For this review, take the finished solid that the model builds, in its own axes (mm). A direction names the side the tool comes from. Round coordinates to 2 decimals unless told otherwise and drop trailing zeros. Write each loop counter-clockwise with the first axis right and the second up, starting at its lowest first coordinate (ties: lowest second). Pieces come first, ordered by that corner, then holes. Notation, with made-up numbers: (38.5, 31.5) -> (71.5, 31.5) arc R21 ccw to (71.5, 67.5) -> close; hole circle Ø9 at (75, -22.75). An arc over 180 degrees is marked (long way). Answer as CSV lines item,"result". Start each with the question number.
Item 1: Mouldability with a two-part tool opening along Z and no side actions: class faces 4 (the flat face through (-31, 1.24, 30)), 5 (the flat face through (44, 1.95, -19)), 6 (the cylindrical face through (-44.339, -1.303, 29.796)), 7 (the flat face through (-44, -2, -7.6)) as +Z half, -Z half, draft (parallel to the pull), parting line (faces both ways), or undercut.
Item 2: Take a section at D-D on y = -3.25. Give the boundary of the cut face in (x, z), then the cut area to 3 significant figures.
Item 3: Take a section at B-B on x = -10. Give the boundary of the cut face in (y, z), then the cut area to 3 significant figures.
Item 4: Wall thickness on probe 1 along X at (y, z) = (-3, 21); probe 2 along Z at (x, y) = (9.5, -1.5); probe 3 along Z at (x, y) = (-20, 2): over which ranges is each line inside the solid? List them lowest first. Write a range as from..to.
Item 5: Take a section at A-A on z = -4. Give the boundary of the cut face in (x, y).
Item 6: Take a section at C-C on z = -19.5. Give the boundary of the cut face in (x, y), then the cut area to 3 significant figures.
Item 7: Machinability: for faces 1 (the flat face through (-44, -2, 7.4)), 2 (the flat face through (-41.05, -3, -17)), 3 (the cylindrical face through (-41.798, 1.232, -27.387)), which of the approach directions +Z, -Z, +X, -X, +Y, -Y give a long, thin tool a straight path to every point of the face, cutting with its end or side? Answer none if there is none.
Item 8: For pin 1 Ø4 at (x, z) = (-33, 30) entering from +Y; pin 2 Ø3 at (x, z) = (44.5, -4.5) entering from +Y; pin 3 Ø1.5 at (y, z) = (-3.5, -1) entering from -X, all flat-tipped, find the tip position at first contact; note any pin that passes through.
```python
from build123d import *

# Parameters (mm, degrees)
EXTRUDE_THIN1_DEPTH      = 2.5
EXTRUDE_THIN1_DEPTH_BACK = 5
EXTRUDE_THIN2_START      = -5
EXTRUDE_THIN2_DEPTH      = 5
CUT_EXTRUDE3_DEPTH       = 76.51403843
CUT_EXTRUDE3_DEPTH_BACK  = 1
CUT_EXTRUDE4_START       = -0.20682878
CUT_EXTRUDE4_OUTLINE_W   = 17
CUT_EXTRUDE4_OUTLINE_H   = 0.9
CUT_EXTRUDE4_OUTLINE_W_2 = 15.6
CUT_EXTRUDE4_OUTLINE_H_2 = 0.55
CUT_EXTRUDE4_DEPTH       = 3.80682878
SKETCH10_W               = 10
SKETCH10_H               = 15
CUT_EXTRUDE6_DEPTH       = 57.113902021
CUT_EXTRUDE11_DEPTH      = 95.199363055
CUT_EXTRUDE11_DEPTH_BACK = 5


# Read off the part's stored shape, not the designer's step: Cut-Extrude4
with BuildPart() as part:
    # Sketch1 → Extrude-Thin1 (new, two sides: drawn at the far end of the back side and taken through both)
    with BuildSketch(Plane(origin=(0, 0, 0), x_dir=(1, 0, 0), z_dir=(0, 1, 0)).offset(-EXTRUDE_THIN1_DEPTH_BACK)):
        with BuildLine():
            Line((-46.05, 25.6), (-46.05, -25.6))
            ThreePointArc((-46.05, -25.6), (-44.292640687, -29.842640687), (-40.05, -31.6))
            Line((-40.05, -31.6), (40.1, -31.6))
            ThreePointArc((40.1, -31.6), (44.342640687, -29.842640687), (46.1, -25.6))
            Line((46.1, -25.6), (46.1, 25.6))
            ThreePointArc((46.1, 25.6), (44.342640687, 29.842640687), (40.1, 31.6))
            Line((40.1, 31.6), (-40.05, 31.6))
            ThreePointArc((-40.05, 31.6), (-44.292640687, 29.842640687), (-46.05, 25.6))
        make_face()
        with BuildLine():
            Line((-42.55, 25.6), (-42.55, -25.6))
            ThreePointArc((-42.55, -25.6), (-41.817766953, -27.367766953), (-40.05, -28.1))
            Line((-40.05, -28.1), (40.1, -28.1))
            ThreePointArc((40.1, -28.1), (41.867766953, -27.367766953), (42.6, -25.6))
            Line((42.6, -25.6), (42.6, 25.6))
            ThreePointArc((42.6, 25.6), (41.867766953, 27.367766953), (40.1, 28.1))
            Line((40.1, 28.1), (-40.05, 28.1))
            ThreePointArc((-40.05, 28.1), (-41.817766953, 27.367766953), (-42.55, 25.6))
        make_face(mode=Mode.SUBTRACT)
    extrude(amount=EXTRUDE_THIN1_DEPTH + EXTRUDE_THIN1_DEPTH_BACK)

    # Sketch1<3> → Extrude-Thin2 (add)
    with BuildSketch(Plane(origin=(0, 0, 0), x_dir=(1, 0, 0), z_dir=(0, 1, 0)).offset(EXTRUDE_THIN2_START)):
        with BuildLine():
            Line((-42.55, 25.6), (-42.55, -25.6))
            ThreePointArc((-42.55, -25.6), (-41.817766953, -27.367766953), (-40.05, -28.1))
            Line((-40.05, -28.1), (40.1, -28.1))
            ThreePointArc((40.1, -28.1), (41.867766953, -27.367766953), (42.6, -25.6))
            Line((42.6, -25.6), (42.6, 25.6))
            ThreePointArc((42.6, 25.6), (41.867766953, 27.367766953), (40.1, 28.1))
            Line((40.1, 28.1), (-40.05, 28.1))
            ThreePointArc((-40.05, 28.1), (-41.817766953, 27.367766953), (-42.55, 25.6))
        make_face()
        with BuildLine():
            Line((-41.05, 25.6), (-41.05, -25.6))
            ThreePointArc((-41.05, -25.6), (-40.757106781, -26.307106781), (-40.05, -26.6))
            Line((-40.05, -26.6), (40.1, -26.6))
            ThreePointArc((40.1, -26.6), (40.807106781, -26.307106781), (41.1, -25.6))
            Line((41.1, -25.6), (41.1, 25.6))
            ThreePointArc((41.1, 25.6), (40.807106781, 26.307106781), (40.1, 26.6))
            Line((40.1, 26.6), (-40.05, 26.6))
            ThreePointArc((-40.05, 26.6), (-40.757106781, 26.307106781), (-41.05, 25.6))
        make_face(mode=Mode.SUBTRACT)
    extrude(amount=EXTRUDE_THIN2_DEPTH)

    # Sketch5 → Cut-Extrude3 (cut, two sides: drawn at the far end of the back side and taken through both)
    with BuildSketch(Plane.XY.offset(28).offset(-CUT_EXTRUDE3_DEPTH_BACK)):
        with BuildLine():
            Line((-26.43, 3.5), (-36.17, 3.5))
            Line((-36.17, 3.5), (-36.17, 2.74))
            ThreePointArc((-36.17, 2.74), (-35.730660172, 1.679339828), (-34.67, 1.24))
            Line((-34.67, 1.24), (-27.93, 1.24))
            ThreePointArc((-27.93, 1.24), (-26.869339828, 1.679339828), (-26.43, 2.74))
            Line((-26.43, 2.74), (-26.43, 3.5))
        make_face()
        with BuildLine():
            Line((-12.954733256, 3.5), (-20.454733256, 3.5))
            Line((-20.454733256, 3.5), (-20.454733256, 3.157106781))
            ThreePointArc((-20.454733256, 3.157106781), (-20.378612788, 2.774423349), (-20.161840037, 2.45))
            Line((-20.161840037, 2.45), (-19.154733256, 1.442893219))
            ThreePointArc((-19.154733256, 1.442893219), (-18.830309907, 1.226120467), (-18.447626475, 1.15))
            Line((-18.447626475, 1.15), (-14.961840037, 1.15))
            ThreePointArc((-14.961840037, 1.15), (-14.579156605, 1.226120467), (-14.254733256, 1.442893219))
            Line((-14.254733256, 1.442893219), (-13.247626475, 2.45))
            ThreePointArc((-13.247626475, 2.45), (-13.030853723, 2.774423349), (-12.954733256, 3.157106781))
            Line((-12.954733256, 3.157106781), (-12.954733256, 3.5))
        make_face()
        with BuildLine():
            Line((0.445266744, 3.5), (-7.054733256, 3.5))
            Line((-7.054733256, 3.5), (-7.054733256, 3.157106781))
            ThreePointArc((-7.054733256, 3.157106781), (-6.978612788, 2.774423349), (-6.761840037, 2.45))
            Line((-6.761840037, 2.45), (-5.754733256, 1.442893219))
            ThreePointArc((-5.754733256, 1.442893219), (-5.430309907, 1.226120467), (-5.047626475, 1.15))
            Line((-5.047626475, 1.15), (-1.561840037, 1.15))
            ThreePointArc((-1.561840037, 1.15), (-1.179156605, 1.226120467), (-0.854733256, 1.442893219))
            Line((-0.854733256, 1.442893219), (0.152373525, 2.45))
            ThreePointArc((0.152373525, 2.45), (0.369146277, 2.774423349), (0.445266744, 3.157106781))
            Line((0.445266744, 3.157106781), (0.445266744, 3.5))
        make_face()
    extrude(amount=CUT_EXTRUDE3_DEPTH + CUT_EXTRUDE3_DEPTH_BACK, mode=Mode.SUBTRACT)

    # Cut-Extrude4 outline → Cut-Extrude4 (cut)
    with BuildSketch(Plane(origin=(42.5, 0, 0), x_dir=(0, 0, -1), z_dir=(1, 0, 0)).offset(CUT_EXTRUDE4_START)):
        with Locations((-17.8, 2.05)):
            Rectangle(CUT_EXTRUDE4_OUTLINE_W, CUT_EXTRUDE4_OUTLINE_H)
        with Locations((19, 2.225)):
            Rectangle(CUT_EXTRUDE4_OUTLINE_W_2, CUT_EXTRUDE4_OUTLINE_H_2)
        with Locations((1.05, 2.225)):
            Rectangle(CUT_EXTRUDE4_OUTLINE_W_2, CUT_EXTRUDE4_OUTLINE_H_2)
    extrude(amount=CUT_EXTRUDE4_DEPTH, mode=Mode.SUBTRACT)

    # Sketch10 → Cut-Extrude6 (cut, through all)
    with BuildSketch(Plane(origin=(0, 0, 0), x_dir=(1, 0, 0), z_dir=(0, 1, 0))):
        with Locations((-46.05, 0.1)):
            Rectangle(SKETCH10_W, SKETCH10_H)
    extrude(amount=-CUT_EXTRUDE6_DEPTH, mode=Mode.SUBTRACT)

    # Sketch11 → Cut-Extrude11 (cut, two sides: drawn at the far end of the back side and taken through both)
    with BuildSketch(Plane.ZY.offset(42.5).offset(-CUT_EXTRUDE11_DEPTH_BACK)):
        with BuildLine():
            ThreePointArc((6.35, 2.5), (6.642893219, 1.792893219), (7.35, 1.5))
            Line((7.35, 1.5), (11.85, 1.5))
            ThreePointArc((11.85, 1.5), (12.557106781, 1.792893219), (12.85, 2.5))
            Line((12.85, 2.5), (6.35, 2.5))
        make_face()
    extrude(amount=CUT_EXTRUDE11_DEPTH + CUT_EXTRUDE11_DEPTH_BACK, mode=Mode.SUBTRACT)


solid = part.part
```
Output values:
1,face 4,"draft"
1,face 5,"undercut"
1,face 6,"+Z half"
1,face 7,"undercut"
2,outline,"(-46.05, -25.6) arc R6 ccw to (-40.05, -31.6) -> (40.1, -31.6) arc R6 ccw to (46.1, -25.6) -> (46.1, 25.6) arc R6 ccw to (40.1, 31.6) -> (-40.05, 31.6) arc R6 ccw to (-46.05, 25.6) -> (-46.05, 7.4) -> (-41.05, 7.4) -> (-41.05, 25.6) arc R1 cw to (-40.05, 26.6) -> (40.1, 26.6) arc R1 cw to (41.1, 25.6) -> (41.1, -25.6) arc R1 cw to (40.1, -26.6) -> (-40.05, -26.6) arc R1 cw to (-41.05, -25.6) -> (-41.05, -7.6) -> (-46.05, -7.6) -> close"
2,area,"1,350 mm^2"
3,outline,"(-5, -31.6) -> (2.5, -31.6) -> (2.5, -28.1) -> (0, -28.1) -> (0, -26.6) -> (-5, -26.6) -> close; (-5, 26.6) -> (0, 26.6) -> (0, 28.1) -> (2.5, 28.1) -> (2.5, 31.6) -> (-5, 31.6) -> close"
3,area,"67.5 mm^2"
4,probe 1,"x = -46.05..-41.05, 41.1..46.1"
4,probe 2,"z = -31.6..-26.6, 26.6..31.6"
4,probe 3,"z = -31.6..-28.1, 28.1..31.6"
5,outline,"(-46.05, 0) -> (-42.55, 0) -> (-42.55, 2.5) -> (-46.05, 2.5) -> close; (41.1, -5) -> (46.1, -5) -> (46.1, 1.95) -> (42.6, 1.95) -> (42.6, 0) -> (41.1, 0) -> close"
6,outline,"(-46.05, -5) -> (-41.05, -5) -> (-41.05, 0) -> (-42.55, 0) -> (-42.55, 2.5) -> (-46.05, 2.5) -> close; (41.1, -5) -> (46.1, -5) -> (46.1, 1.95) -> (42.6, 1.95) -> (42.6, 0) -> (41.1, 0) -> close"
6,area,"65.6 mm^2"
7,face 1,"-X, -Y"
7,face 2,"+Y, -Y"
7,face 3,"+Y"
8,pin 1,"stops at y = 1.28"
8,pin 2,"stops at y = 1.95"
8,pin 3,"stops at x = 41.1"
